Design review of the part built by this model. Coordinates are the model's own, in mm. Face numbers are marked on the shaded views. A direction names the side the tool comes from. Coordinates: 2 decimals unless noted, no trailing zeros. Write each loop counter-clockwise with the first axis right and the second up, starting at its lowest first coordinate (ties: lowest second). Pieces come first, ordered by that corner, then holes. Notation, with made-up numbers: M -2,15 L 13,15 A23 ccw 13,38 Z; hole C -31.5,69.25 d1. An arc over 180 degrees is marked long. Write each question's results on one line, items separated by ' | '. Start each with the question number.
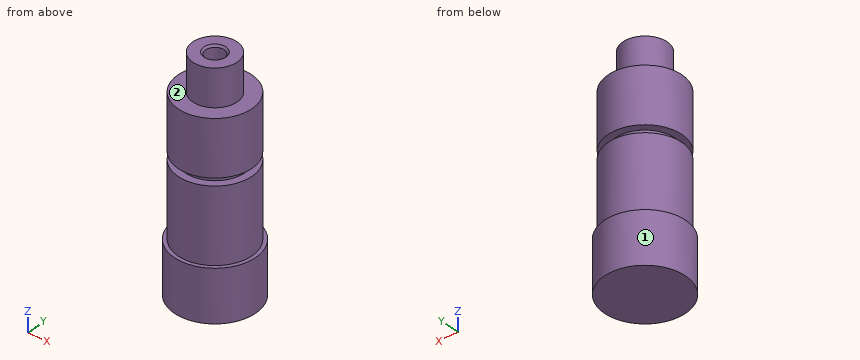
```python
from build123d import *

# Parameters (mm, degrees)
ESQUISSE1_R                     = 11
BASE_EXTRUSION_DEPTH            = 14
ESQUISSE2_R                     = 10
BOSS_EXTRU_1_DEPTH              = 37
ESQUISSE3_W                     = 2
ESQUISSE3_H                     = 2
ESQUISSE4_R                     = 6
BOSS_EXTRU_2_DEPTH              = 10
TROU_TARAUD_M6X1_01_D           = 5
TROU_TARAUD_M6X1_01_DEPTH       = 19
TROU_TARAUD_M6X1_01_CSINK_D     = 6
TROU_TARAUD_M6X1_01_CSINK_ANGLE = 90
TROU_TARAUD_M6X1_01_TIP         = 1.502151548


with BuildPart() as part:
    # Esquisse1 → Base-Extrusion (new body)
    with BuildSketch(Plane.XY):
        Circle(ESQUISSE1_R)
    extrude(amount=BASE_EXTRUSION_DEPTH)

    # Esquisse2 → Boss.-Extru.1 (add)
    with BuildSketch(Plane.XY.offset(14)):
        with Locations(Location((0, 0, 0), (0, 0, 180))):
            Circle(ESQUISSE2_R)
    extrude(amount=BOSS_EXTRU_1_DEPTH)

    # Esquisse3 → Enlèvement de matière-Révolution1 (revolve, cut)
    with BuildSketch(Plane(origin=(0, 0, 0), x_dir=(1, 0, 0), z_dir=(0, 1, 0))):
        with Locations((9, -35)):
            Rectangle(ESQUISSE3_W, ESQUISSE3_H)
    revolve(axis=Axis((0, 0, 0), (0, 0, 1)), mode=Mode.SUBTRACT)

    # Esquisse4 → Boss.-Extru.2 (add)
    with BuildSketch(Plane.XY.offset(51)):
        Circle(ESQUISSE4_R)
    extrude(amount=BOSS_EXTRU_2_DEPTH)

    # Trou taraudé M6x1.01
    with Locations(Plane.XY.offset(61)):
        with Locations((0, 0)):
            CounterSinkHole(TROU_TARAUD_M6X1_01_D / 2, TROU_TARAUD_M6X1_01_CSINK_D / 2, depth=TROU_TARAUD_M6X1_01_DEPTH, counter_sink_angle=TROU_TARAUD_M6X1_01_CSINK_ANGLE)
            with Locations((0, 0, -(TROU_TARAUD_M6X1_01_DEPTH + TROU_TARAUD_M6X1_01_TIP / 2))):  # 118° drill point
                Cone(0, TROU_TARAUD_M6X1_01_D / 2, TROU_TARAUD_M6X1_01_TIP, mode=Mode.SUBTRACT)


solid = part.part
```
Item 1: Insertion check: pin 1 Ø5 at (x, z) = (5, 32.5) entering from -Y; pin 2 Ø1 at (x, z) = (5, 20.5) entering from +Y; pin 3 Ø1.5 at (x, z) = (-0.5, 37) entering from +Y. Each pin has a flat end and moves straight along its axis. Give the tip position at first contact, or say it passes through.
Item 2: For the marked faces 1 and 2, list the 3-axis set-ups (+Z, -Z, +X, -X, +Y, -Y) from which the entire face can be reached by the end or side of a thin tool; tool diameter is ignored.
Item 3: We need section B-B on x = -7. State the section outline as (y, z) points, then the cut area to 3 significant figures.
Item 4: We need section C-C on y = -5. State the section outline as (x, z) points (3 decimals), then the cut area to 3 significant figures.
Item 5: Wall thickness on L1, parallel to Y at x = 0, z = 51.25; L2, parallel to Y at x = 0, z = 48; L3, parallel to Z at x = 1.25, y = -8.75: over which ranges is each line inside the solid? List them lowest first.
Item 6: We need section A-A on z = 45.5. State the section outline as (x, y) points.
Item 7: We need section D-D on z = 23. State the section outline as (x, y) points.
Answer:
1) pin 1: stops at y = -9.68 | pin 2: stops at y = 8.93 | pin 3: stops at y = 10
2) face 1: +Z, -Z | face 2: +Z
3) outline: M -8.49,0 L 8.49,0 L 8.49,14 L 7.14,14 L 7.14,34 L 3.87,34 L 3.87,36 L 7.14,36 L 7.14,51 L -7.14,51 L -7.14,36 L -3.87,36 L -3.87,34 L -7.14,34 L -7.14,14 L -8.49,14 Z | area: 753 mm^2
4) outline: M -9.798,0 L 9.798,0 L 9.798,14 L 8.66,14 L 8.66,34 L 6.245,34 L 6.245,36 L 8.66,36 L 8.66,51 L 3.317,51 L 3.317,61 L -3.317,61 L -3.317,51 L -8.66,51 L -8.66,36 L -6.245,36 L -6.245,34 L -8.66,34 L -8.66,14 L -9.798,14 Z | area: 972 mm^2
5) L1: y = -6 to -2.5, 2.5 to 6 | L2: y = -10 to -2.5, 2.5 to 10 | L3: z = 0 to 34, 36 to 51
6) outline: C 0,0 d20; hole C 0,0 d5
7) outline: C 0,0 d20
